Verification items for this drawing (mm, ordinates from the low corner). A direction names the side the tool comes from. Coordinates: 2 decimals unless noted, no trailing zeros. Order: outer loops, then holes, each group sorted by start corner. A loop starts at its lowest first (then second) coordinate and runs counter-clockwise, first axis right, second up. Notation, with made-up numbers: (40, 16.25) -> (47, 16.25) arc R28 ccw to (47, 46.25) -> close; hole circle Ø1 at (52.25, 71.25). An arc over 180 degrees is marked (long way). Write item = value, one per line. Start each with the question number.
1. Thickness scan on line 1 along Y through (x, z) = (5, 2.8); line 2 along Z through (x, y) = (4.5, 13); line 3 along Y through (x, z) = (6.25, 7.25). Record the ranges inside material, lowest first. Write a range as from..to.
2. Go/stop test with flat-tipped pins: P1, Ø4, axis at y = 3.5, z = 6.5, coming from the -X side; P2, Ø1, axis at x = 8.5, y = 14.5, coming from the +Z side; P3, Ø1, axis at x = 12, z = 0.5, coming from the -Y side. Record where each tip stops, or that it passes through.
3. Release check for a two-part mould opening along Y. For the marked faces 6, 7 and 8 record: +Y half, -Y half, draft (parallel to the pull), parting line (faces both ways), or undercut.
4. Cross-section at B-B on y = 18. Record the cut outline in (x, z), plus the area to 3 significant figures.
5. Cross-section at C-C on y = 23.75. Record the cut outline in (x, z), plus the area to 3 significant figures.
6. Cross-section at D-D on x = 9.75. Record the cut outline in (y, z), plus the area to 3 significant figures.
7. Cross-section at A-A on x = 5. Record the cut outline in (y, z).
8. Set-up check for the marked faces 1, 2, 3, 4 and 5: record each of +Z, -Z, +X, -X, +Y, -Y from which the full face is reachable in a straight line by a thin tool's end or side.
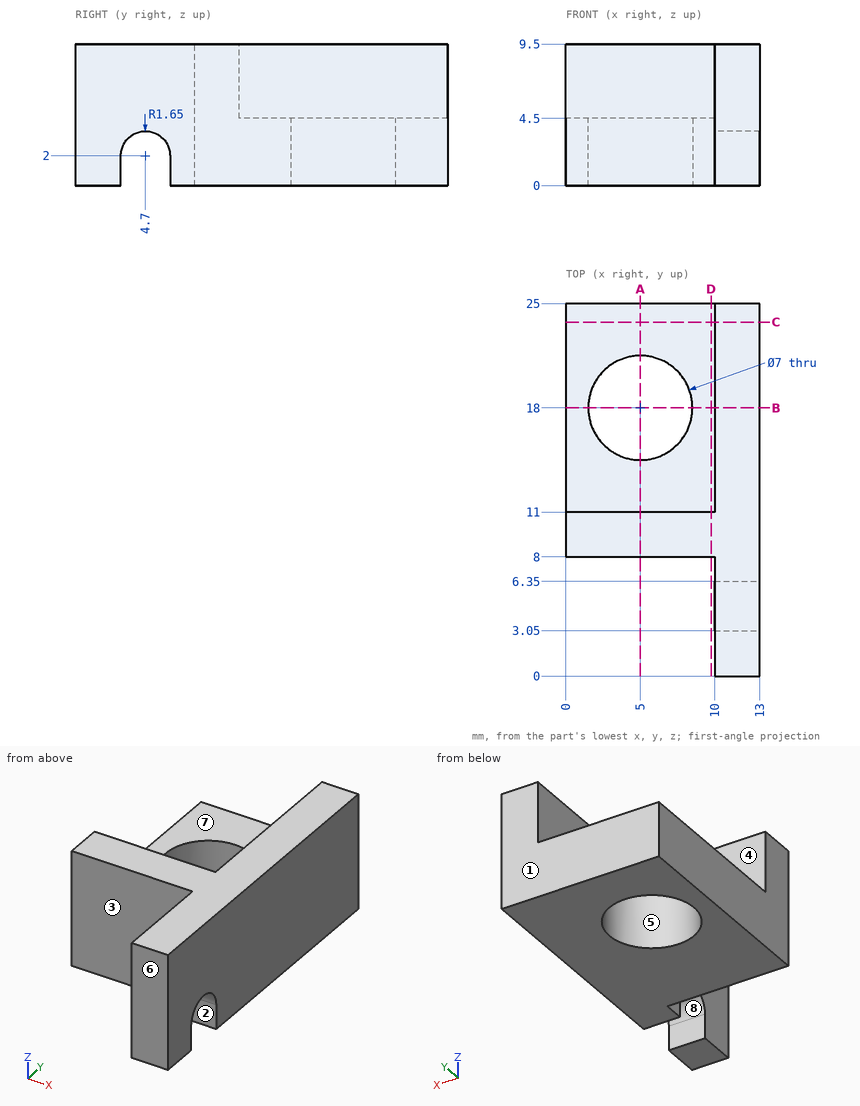
Worked out:
q1.line_1 = 8..14.5, 21.5..25
q1.line_2 = 0..4.5
q1.line_3 = 8..11
q2.P1 = 10
q2.P2 = 4.5
q2.P3 = 0
q3.face_6 = -Y half
q3.face_7 = draft
q3.face_8 = undercut
q4.outline = (0, 0) -> (1.5, 0) -> (1.5, 4.5) -> (0, 4.5) -> close; (8.5, 0) -> (13, 0) -> (13, 9.5) -> (10, 9.5) -> (10, 4.5) -> (8.5, 4.5) -> close
q4.area = 42.0 mm²
q5.outline = (0, 0) -> (13, 0) -> (13, 9.5) -> (10, 9.5) -> (10, 4.5) -> (0, 4.5) -> close
q5.area = 73.5 mm²
q6.outline = (8, 0) -> (25, 0) -> (25, 4.5) -> (11, 4.5) -> (11, 9.5) -> (8, 9.5) -> close
q6.area = 91.5 mm²
q7.outline = (8, 0) -> (14.5, 0) -> (14.5, 4.5) -> (11, 4.5) -> (11, 9.5) -> (8, 9.5) -> close; (21.5, 0) -> (25, 0) -> (25, 4.5) -> (21.5, 4.5) -> close
q8.face_1 = +Z, -Z, +X, -X, +Y
q8.face_2 = -Z, +X, -X
q8.face_3 = +Z, -Z, -X, -Y
q8.face_4 = +Z, -X, +Y
q8.face_5 = +Z, -Z
